The listing builds one solid part. Answer for the finished solid, in the listing's coordinates (mm). A direction names the side the tool comes from. Give positions to 0.01 mm unless a question says otherwise; leave off trailing zeros. Write each loop counter-clockwise with the first axis right and the second up, starting at its lowest first coordinate (ties: lowest second). Pieces come first, ordered by that corner, then holes. Notation, with made-up numbers: (18.5, -38.5) - (46.5, -38.5) arc R13 ccw to (46.5, -16.5) - close; hole circle Ø1 at (75, 45). An arc over 180 degrees is marked (long way). One line per question, with ' | ' between items. Start each with the question number.
1. The mould has two halves that part along Z. Classify faces 6 (the face through (2, -6, 11.4)), 7 (the face through (1.9, -21, 25.2)), 8 (the face through (2, -6, 24.4)), 9 (the face through (15.23, -20.72, 5.29)): +Z half, -Z half, draft (parallel to the pull), parting line (faces both ways), or undercut.
2. Find the intervals of material crossed by L1, parallel to Y at x = 1.5, z = 17.9; L2, parallel to Y at x = -0.5, z = 17.9; L3, parallel to Z at x = 13.5, y = 5, in increasing order. Write a range as from..to.
3. A cutting plane is placed at D-D (z = 18.25). State how many separate pieces and enclosed holes the cut face has, then the cut area to 3 significant figures.
4. A cutting plane is placed at C-C (y = -15.5). Determine the outline of the cut face in (x, z), then the cut area to 3 significant figures.
5. Given P1, Ø2.5, axis at y = -19.3, z = 17.9, coming from the +X side; P2, Ø1, axis at y = -19.5, z = 18.5, coming from the -X side; P3, Ø0.8, axis at y = -4.5, z = 5.5, coming from the +X side, each flat-ended and moving along its own axis, determine where each tip first touches the part or whether it passes through.
6. For faces 1 (the face through (2, 5.9, 18)), 2 (the face through (3.5, -1, 26)), 3 (the face through (11.896, -15.193, 5.289)), 4 (the face through (-0.686, 8.876, 18.117)), 5 (the face through (-1.7, -19.3, 16.7)), determine the directions among +Z, -Z, +X, -X, +Y, -Y from which every point of the face is accessible in a straight line to the end or side of a thin tool.
7. A cutting plane is placed at A-A (y = -5.5). Determine the outline of the cut face in (x, z), then the cut area to 3 significant figures.
8. A cutting plane is placed at B-B (x = -20). Determine the outline of the cut face in (y, z), then the cut area to 3 significant figures.
```python
from build123d import *

# Parameters (mm, degrees)
PAD002_DEPTH    = 34
SKETCH003_R     = 0.9
POCKET001_DEPTH = 22.001
SKETCH005_W     = 13
SKETCH005_H     = 23.2
POCKET002_DEPTH = 22.001
SKETCH006_R     = 1.25
PAD003_DEPTH    = 1.6
SKETCH007_R     = 1.25
PAD004_DEPTH    = 1.6
SKETCH009_R     = 1.8
SKETCH009_R_2   = 1
PAD005_DEPTH    = 2
CHAMFER_SIZE    = 3
CHAMFER001_SIZE = 12


with BuildPart() as part:
    # Sketch004 → Pad002 (new body)
    with BuildSketch(Plane.XZ):
        Polygon((-22, 1.6), (-8.2, 1.6), (-3.2, 6.6), (-3.2, 22.2), (0, 22.2), (0, 6.6), (4, 1.6), (4, 0), (-3.601763, 0), (-22, 0), align=None)
    extrude(amount=PAD002_DEPTH)

    # Sketch003 → Pocket001 (cut, through all)
    with BuildSketch(Plane(origin=(0, 0, 0), x_dir=(0, 0, 1), z_dir=(1, 0, 0))):
        with Locations((13.4, 30.8)):
            Circle(SKETCH003_R)
        with Locations((13.4, 3.6)):
            Circle(SKETCH003_R)
    extrude(amount=-POCKET001_DEPTH, mode=Mode.SUBTRACT)

    # Sketch005 (on DatumPlane) → Pocket002 (cut, through all)
    with BuildSketch(Plane(origin=(0, 0, 0), x_dir=(0, 0, 1), z_dir=(1, 0, 0))):
        with Locations((13.4, 17.2)):
            Rectangle(SKETCH005_W, SKETCH005_H)
    extrude(amount=-POCKET002_DEPTH, mode=Mode.SUBTRACT)

    # Sketch006 → Pad003 (join)
    with BuildSketch(Plane.XY):
        with BuildLine():
            ThreePointArc((-24.911765, -14.352941), (-26.5, -17), (-24.911765, -19.647059))
            Line((-20.5, -22), (-24.911765, -19.647059))
            Line((-20.5, -12), (-20.5, -22))
            Line((-20.5, -12), (-24.911765, -14.352941))
        make_face()
        with Locations((-23.5, -17)):
            Circle(SKETCH006_R, mode=Mode.SUBTRACT)
    extrude(amount=PAD003_DEPTH)

    # Sketch007 → Pad004 (join)
    with BuildSketch(Plane.XY):
        with BuildLine():
            ThreePointArc((12, -34), (14.963938, -31.463756), (12.916362, -28.143379))
            Line((0, -24), (12.916362, -28.143379))
            Line((0, -34), (0, -24))
            Line((0, -34), (12, -34))
        make_face()
        with Locations((12, -31)):
            Circle(SKETCH007_R, mode=Mode.SUBTRACT)
        with BuildLine():
            ThreePointArc((12.916362, -5.856621), (14.96394, -2.536256), (12.000023, 0))
            Line((0, 0), (12.000023, 0))
            Line((0, 0), (0, -10))
            Line((0, -10), (12.916362, -5.856621))
        make_face()
        with Locations((12, -3)):
            Circle(SKETCH007_R, mode=Mode.SUBTRACT)
    extrude(amount=PAD004_DEPTH)

    # Sketch009 (on Face2 of Pad004) → Pad005 (join)
    with BuildSketch(Plane(origin=(-3.2, 0, 0), x_dir=(0, 0, -1), z_dir=(-1, 0, 0))):
        with Locations((-13.4, 30.8)):
            Circle(SKETCH009_R)
        with Locations((-13.4, 30.8)):
            Circle(SKETCH009_R_2, mode=Mode.SUBTRACT)
        with Locations((-13.4, 3.6)):
            Circle(SKETCH009_R)
        with Locations((-13.4, 3.6)):
            Circle(SKETCH009_R_2, mode=Mode.SUBTRACT)
    extrude(amount=PAD005_DEPTH)

    # Chamfer
    chamfer_edges = [part.edges().sort_by_distance(p)[0] for p in [
        (-1.6, -34, 22.2),
        (-1.6, 0, 22.2),
    ]]
    chamfer(chamfer_edges, length=CHAMFER_SIZE)

    # Chamfer001
    chamfer001_edges = [part.edges().sort_by_distance(p)[0] for p in [
        (-22, -34, 0.8),
        (-22, 0, 0.8),
    ]]
    chamfer(chamfer001_edges, length=CHAMFER001_SIZE)


with BuildPart() as part_1:
    # Body001 placement: moved
    add(part.part.moved(Location((3.5, 11.5, 4.5))))


solid = part_1.part
```
Determined:
1) face 6: undercut | face 7: +Z half | face 8: undercut | face 9: draft
2) L1: -22.5..-20.2, -18.4..-17.3, 5.9..7, 8.8..11.5 | L2: -21.1..-20.3, -18.3..-17.5, 6.1..6.9, 8.9..9.7 | L3: 4.5..6.1
3) separate pieces: 4 | enclosed holes: 0 | area: 30.6 mm2
4) outline: (-13.5, 4.5) - (12.85, 4.5) - (12.85, 6.1) - (7.5, 6.1) - (3.5, 11.1) - (3.5, 11.4) - (0.3, 11.4) - (0.3, 11.1) - (-4.7, 6.1) - (-13.5, 6.1) - close; (0.3, 24.4) - (3.5, 24.4) - (3.5, 26.7) - (0.3, 26.7) - close | area: 89.0 mm2
5) P1: x = 3.5 | P2: x = -1.7 | P3: x = 7.5
6) face 1: +X, -X | face 2: +Z, +X, +Y, -Y | face 3: +Z, -Z, +X | face 4: -X | face 5: +Z, -X, +Y, -Y
7) outline: (-23, 4.5) - (-21.25, 4.5) - (-21.25, 6.1) - (-23, 6.1) - close; (-18.75, 4.5) - (7.5, 4.5) - (7.5, 6.1) - (3.5, 11.1) - (3.5, 11.4) - (0.3, 11.4) - (0.3, 11.1) - (-4.7, 6.1) - (-18.75, 6.1) - close; (0.3, 24.4) - (3.5, 24.4) - (3.5, 26.7) - (0.3, 26.7) - close | area: 91.6 mm2
8) outline: (-8.9, 4.5) - (-6.75, 4.5) - (-6.75, 6.1) - (-8.9, 6.1) - close; (-4.25, 4.5) - (-2.1, 4.5) - (-2.1, 6.1) - (-4.25, 6.1) - close | area: 6.88 mm2
